Can you work these out from the model? Positions are in its coordinate system, mm. A direction names the side the tool comes from. Coordinates: 2 decimals unless noted, no trailing zeros. Order: outer loops, then holes, each group sorted by start corner. A loop starts at its lowest first (then second) coordinate and runs counter-clockwise, first axis right, second up. Notation, with made-up numbers: M 79,16 L 94,16 A33 cw 94,51 Z; hole C 6,83.5 d1. An arc over 180 degrees is marked long. Answer as CSV lines item,"result". Start each with the question number.
1. If we section it at A-A (x = 28.5): List the corners of the cut face in (y, z) for me.
2. Will these pins go through, and if not, where does the flat tip stop? pin 1 (3 mm diameter, centred on y = 1, z = -12, fed in from +X); pin 2 (3 mm diameter, centred on x = -9.5, z = -10, fed in from +Y); pin 3 (1.5 mm diameter, centred on x = -30, y = 1, fed in from -Z).
3. If we section it at B-B (z = -4): List the corners of the cut face in (x, y) for me.
4. If we section it at C-C (x = 10): List the corners of the cut face in (y, z) for me (3 decimals).
5. On a 3-axis mill with a long thin cutter (end or side, diameter ignored), from which of +Z, -Z, +X, -X, +Y, -Y can I reach the whole of each face in a straight line? I mean faces 1 (the face through (-8.6, 1.6, -11.4)), 2 (the face through (46.076, 1.16, 13.607)). Say none if no direction works.
6. I need wall thicknesses on line 1 along Z through (x, y) = (28.5, 3.2); line 2 along X through (y, z) = (4.2, 8.5); line 3 along X through (y, z) = (2.15, 8.5). Which ranges of each line are inside material? Lowest first, please. Write a range as from..to.
7. If we mould it in two halves opening along X, with no side actions, what happens to faces 3 (the face through (-47, 1.5, 0.2)), 4 (the face through (-1, 2, -15)), 5 (the face through (11.4, 1.6, 8.6)), 6 (the face through (46.118, 1.202, -13.649))? For each: released by +X, released by -X, zero draft, split by the parting line, or undercut.
8. If we section it at D-D (x = -23): List the corners of the cut face in (y, z) for me, plus the area to 3 significant figures.
```python
from build123d import *

# Parameters (mm, degrees)
SKETCH1_W                                    = 97
SKETCH1_H                                    = 32
BOSS_EXTRUDE1_DEPTH                          = 5
HOLE1_D                                      = 4.5
HOLE1_DEPTH                                  = 6
CHAMFER1_SIZE                                = 1
CHAMFER2_SIZE                                = 3
FILLET1_R                                    = 3
CBORE_FOR_M3_HEX_SOCKET_HEAD_CAP_SCR_2_COUNT = 2
CBORE_FOR_M3_HEX_SOCKET_HEAD_CAP_SCR_2_PITCH = 20
CBORE_FOR_M3_HEX_SOCKET_HEAD_CAP_SCR_3_COUNT = 2
CBORE_FOR_M3_HEX_SOCKET_HEAD_CAP_SCR_3_PITCH = 20
CBORE_FOR_M3_HEX_SOCKET_HEAD_CAP_SCR_4_COUNT = 2
CBORE_FOR_M3_HEX_SOCKET_HEAD_CAP_SCR_4_PITCH = 28.284271247


with BuildPart() as part:
    # Sketch1 → Boss-Extrude1 (new body)
    with BuildSketch(Plane(origin=(0, 0, 0), x_dir=(1, 0, 0), z_dir=(0, 1, 0))):
        Rectangle(SKETCH1_W, SKETCH1_H)
    extrude(amount=BOSS_EXTRUDE1_DEPTH)

    # Hole1
    with Locations(Plane(origin=(0, 5, 0), x_dir=(1, 0, 0), z_dir=(0, 1, 0))):
        with Locations((-28.5, 8.5), (-28.5, -8.5), (28.5, -8.5), (28.5, 8.5)):
            Hole(HOLE1_D / 2, depth=HOLE1_DEPTH)

    # Chamfer1
    chamfer1_edges = [part.edges().sort_by_distance(p)[0] for p in [
        (-48.5, 5, 0),
        (0, 5, 16),
        (48.5, 5, 0),
        (0, 5, -16),
    ]]
    chamfer(chamfer1_edges, length=CHAMFER1_SIZE)

    # Chamfer2
    chamfer2_edges = [part.edges().sort_by_distance(p)[0] for p in [
        (0, 0, 16),
        (-48.5, 0, 0),
        (0, 0, -16),
        (48.5, 0, 0),
    ]]
    chamfer(chamfer2_edges, length=CHAMFER2_SIZE)

    # Fillet1
    # the kernel refuses this fillet: 3 mm, written as the material it takes off along each edge
    with BuildSketch(Plane(origin=(48.5, -4.5, 16), x_dir=(0, 0, -1), z_dir=(0, 1, 0)), Plane(origin=(48.5, -4.5, -16), x_dir=(-1, 0, 0), z_dir=(0, 1, 0))) as fillet1_piece_1:
        with BuildLine():
            CenterArc((FILLET1_R, FILLET1_R), FILLET1_R, 180, 90)
            Line((0, FILLET1_R), (0, 0))
            Line((0, 0), (FILLET1_R, 0))
        make_face()
    extrude(amount=16, mode=Mode.SUBTRACT)
    with BuildSketch(Plane(origin=(-48.5, -4.5, 16), x_dir=(0, 0, -1), z_dir=(0, 1, 0)), Plane(origin=(-48.5, -4.5, -16), x_dir=(1, 0, 0), z_dir=(0, 1, 0))) as fillet1_piece_2:
        with BuildLine():
            CenterArc((FILLET1_R, -FILLET1_R), FILLET1_R, 90, 90)
            Line((0, -FILLET1_R), (0, 0))
            Line((0, 0), (FILLET1_R, 0))
        make_face()
    extrude(amount=16, mode=Mode.SUBTRACT)
    with BuildSketch(Plane(origin=(-51, 1.5, -18.5), x_dir=(0.8164965809277261, -0.40824829046386363, -0.40824829046386235), z_dir=(0.5773502691896258, 0.5773502691896258, 0.5773502691896258)), Plane(origin=(-51, 1.5, 18.5), x_dir=(-0.4082482904638625, -0.4082482904638635, -0.8164965809277259), z_dir=(0.5773502691896258, 0.5773502691896258, -0.5773502691896258)), Plane(origin=(45, 7.5, 12.5), x_dir=(0.40824829046386274, -0.40824829046386324, -0.816496580927726), z_dir=(0.5773502691896258, -0.5773502691896258, 0.5773502691896258))) as fillet1_piece_3:
        with BuildLine():
            CenterArc((FILLET1_R * 0.57735026919, -FILLET1_R), FILLET1_R, 90, 60)
            Line((-FILLET1_R * 0.288675134595, -FILLET1_R * 0.5), (0, 0))
            Line((0, 0), (FILLET1_R * 0.57735026919, 0))
        make_face()
    extrude(amount=10.392304845, mode=Mode.SUBTRACT)
    with BuildSketch(Plane(origin=(51, 1.5, -18.5), x_dir=(-0.816496580927726, -0.4082482904638631, -0.40824829046386285), z_dir=(-0.5773502691896258, 0.5773502691896258, 0.5773502691896258))) as fillet1_piece_4:
        with BuildLine():
            CenterArc((FILLET1_R * 0.57735026919, FILLET1_R), FILLET1_R, 210, 60)
            Line((-FILLET1_R * 0.288675134595, FILLET1_R * 0.5), (0, 0))
            Line((0, 0), (FILLET1_R * 0.57735026919, 0))
        make_face()
    extrude(amount=10.392304845, mode=Mode.SUBTRACT)
    with BuildSketch(Plane(origin=(-43, -2.5, 10.5), x_dir=(-0.4082482904638623, 0.4082482904638638, -0.816496580927726), z_dir=(-0.5773502691896258, 0.5773502691896258, 0.5773502691896258)), Plane(origin=(51, 5.5, -18.5), x_dir=(-0.816496580927726, 0.40824829046386324, -0.40824829046386274), z_dir=(-0.5773502691896258, -0.5773502691896258, 0.5773502691896258))) as fillet1_piece_5:
        with BuildLine():
            CenterArc((FILLET1_R * 0.57735026919, -FILLET1_R), FILLET1_R, 90, 60)
            Line((-FILLET1_R * 0.288675134595, -FILLET1_R * 0.5), (0, 0))
            Line((0, 0), (FILLET1_R * 0.57735026919, 0))
        make_face()
    extrude(amount=13.856406461, mode=Mode.SUBTRACT)
    with BuildSketch(Plane(origin=(-51, 5.5, -18.5), x_dir=(0.816496580927726, 0.4082482904638625, -0.4082482904638635), z_dir=(0.5773502691896258, -0.5773502691896258, 0.5773502691896258)), Plane(origin=(43, -2.5, 10.5), x_dir=(0.40824829046386285, 0.40824829046386313, -0.816496580927726), z_dir=(0.5773502691896258, 0.5773502691896258, 0.5773502691896258))) as fillet1_piece_6:
        with BuildLine():
            CenterArc((FILLET1_R * 0.57735026919, FILLET1_R), FILLET1_R, 210, 60)
            Line((-FILLET1_R * 0.288675134595, FILLET1_R * 0.5), (0, 0))
            Line((0, 0), (FILLET1_R * 0.57735026919, 0))
        make_face()
    extrude(amount=13.856406461, mode=Mode.SUBTRACT)

    # Sketch7 → CBORE for M3 Hex Socket Head Cap Screw1 (revolve, cut)
    with BuildSketch(Plane(origin=(10, 5, -10), x_dir=(0, 0, 1), z_dir=(1, 0, 0))):
        Polygon((0, 0), (0, 5), (1.7, 5), (1.7, 3.4), (3.25, 3.4), (3.25, 0.025), (3.275, 0), align=None)
    cbore_for_m3_hex_socket_head_cap_screw1 = revolve(axis=Axis((10, 11.35, -10), (0, -1, 0)), mode=Mode.SUBTRACT)

    # CBORE for M3 Hex Socket Head Cap Scr 2: CBORE for M3 Hex Socket Head Cap Screw1 ×2
    with Locations(*[(-i * CBORE_FOR_M3_HEX_SOCKET_HEAD_CAP_SCR_2_PITCH, 0, 0) for i in range(1, CBORE_FOR_M3_HEX_SOCKET_HEAD_CAP_SCR_2_COUNT)]):
        add(cbore_for_m3_hex_socket_head_cap_screw1, mode=Mode.SUBTRACT)

    # CBORE for M3 Hex Socket Head Cap Scr 3: CBORE for M3 Hex Socket Head Cap Screw1 ×2
    with Locations(*[(0, 0, i * CBORE_FOR_M3_HEX_SOCKET_HEAD_CAP_SCR_3_PITCH) for i in range(1, CBORE_FOR_M3_HEX_SOCKET_HEAD_CAP_SCR_3_COUNT)]):
        add(cbore_for_m3_hex_socket_head_cap_screw1, mode=Mode.SUBTRACT)

    # CBORE for M3 Hex Socket Head Cap Scr 4: CBORE for M3 Hex Socket Head Cap Screw1 ×2
    with Locations(*[Vector(-0.7071067811865475, 0, 0.7071067811865477) * (i * CBORE_FOR_M3_HEX_SOCKET_HEAD_CAP_SCR_4_PITCH) for i in range(1, CBORE_FOR_M3_HEX_SOCKET_HEAD_CAP_SCR_4_COUNT)]):
        add(cbore_for_m3_hex_socket_head_cap_screw1, mode=Mode.SUBTRACT)


solid = part.part
```
Solved:
1,outline,"M 0,-13 L 3,-16 L 4,-16 L 5,-15 L 5,-10.75 L 0,-10.75 Z; M 0,-6.25 L 5,-6.25 L 5,6.25 L 0,6.25 Z; M 0,10.75 L 5,10.75 L 5,15 L 4,16 L 3,16 L 0,13 Z"
2,pin 1,"x = 48"
2,pin 2,"y = 1.6"
2,pin 3,"z = -14.75"
3,outline,"M -48.5,3 L -45.5,0 L 45.5,0 L 48.5,3 L 48.5,4 L 47.5,5 L -47.5,5 L -48.5,4 Z"
4,outline,"M 0,-13 L 3,-16 L 4,-16 L 5,-15 L 5,-13.275 L 4.975,-13.25 L 1.6,-13.25 L 1.6,-11.7 L 0,-11.7 Z; M 0,-8.3 L 1.6,-8.3 L 1.6,-6.75 L 4.975,-6.75 L 5,-6.725 L 5,6.725 L 4.975,6.75 L 1.6,6.75 L 1.6,8.3 L 0,8.3 Z; M 0,11.7 L 1.6,11.7 L 1.6,13.25 L 4.975,13.25 L 5,13.275 L 5,15 L 4,16 L 3,16 L 0,13 Z"
5,face 1,"+Y"
5,face 2,"+Z, +X, -Y"
6,line 1,"-16..-10.75, -6.25..6.25, 10.75..16"
6,line 2,"-48.3..-30.75, -26.25..-12.88, -7.12..7.12, 12.88..26.25, 30.75..48.3"
6,line 3,"-47.65..-30.75, -26.25..-12.88, -7.12..7.12, 12.88..26.25, 30.75..47.65"
7,face 3,"released by -X"
7,face 4,"zero draft"
7,face 5,"undercut"
7,face 6,"released by +X"
8,outline,"M 0,-13 L 3,-16 L 4,-16 L 5,-15 L 5,15 L 4,16 L 3,16 L 0,13 Z"
8,area,"150 mm²"
